```python
from build123d import *

# Parameters (mm, degrees)
SKETCH1_W                         = 78
SKETCH1_H                         = 60
BOSS_EXTRUDE1_DEPTH               = 9.3
TAP_DRILL_FOR_M5_TAP1_D           = 5.2
TAP_DRILL_FOR_M5_TAP1_DEPTH       = 46
TAP_DRILL_FOR_M5_TAP1_CSINK_D     = 6
TAP_DRILL_FOR_M5_TAP1_CSINK_ANGLE = 90
TAP_DRILL_FOR_M5_TAP1_TIP         = 1.562237609
SKETCH4_W                         = 61.6
SKETCH4_H                         = 60
CUT_EXTRUDE1_DEPTH                = 5.3
CHAMFER1_SIZE                     = 3
CUT_EXTRUDE2_DEPTH                = 4
FILLET1_R                         = 1
FILLET2_R                         = 1
SKETCH7_W                         = 8
SKETCH7_H                         = 20
BOSS_EXTRUDE2_DEPTH               = 5.3
SKETCH8_R                         = 1.75
CUT_EXTRUDE3_DEPTH                = 5.3


with BuildPart() as part:
    # Sketch1 → Boss-Extrude1 (new body)
    with BuildSketch(Plane(origin=(0, 0, 0), x_dir=(1, 0, 0), z_dir=(0, 1, 0))):
        Rectangle(SKETCH1_W, SKETCH1_H)
    extrude(amount=BOSS_EXTRUDE1_DEPTH)

    # Tap Drill for M5 Tap1
    with Locations(Plane(origin=(-36, 9.3, -15), x_dir=(0, 0, 1), z_dir=(0, 1, 0))):
        with Locations((0, 0), (30, 0), (30, 72), (0, 72)):
            CounterSinkHole(TAP_DRILL_FOR_M5_TAP1_D / 2, TAP_DRILL_FOR_M5_TAP1_CSINK_D / 2, depth=TAP_DRILL_FOR_M5_TAP1_DEPTH, counter_sink_angle=TAP_DRILL_FOR_M5_TAP1_CSINK_ANGLE)
            with Locations((0, 0, -(TAP_DRILL_FOR_M5_TAP1_DEPTH + TAP_DRILL_FOR_M5_TAP1_TIP / 2))):  # 118° drill point
                Cone(0, TAP_DRILL_FOR_M5_TAP1_D / 2, TAP_DRILL_FOR_M5_TAP1_TIP, mode=Mode.SUBTRACT)

    # Sketch4 → Cut-Extrude1 (cut)
    with BuildSketch(Plane(origin=(0, 9.3, 0), x_dir=(1, 0, 0), z_dir=(0, 1, 0))):
        Rectangle(SKETCH4_W, SKETCH4_H)
    extrude(amount=-CUT_EXTRUDE1_DEPTH, mode=Mode.SUBTRACT)

    # Chamfer1
    chamfer1_edges = [part.edges().sort_by_distance(p)[0] for p in [
        (39, 4.65, 30),
        (-39, 4.65, 30),
        (-39, 4.65, -30),
        (39, 4.65, -30),
    ]]
    chamfer(chamfer1_edges, length=CHAMFER1_SIZE)

    # Sketch6 → Cut-Extrude2 (cut)
    with BuildSketch(Plane(origin=(0, 9.3, 0), x_dir=(1, 0, 0), z_dir=(0, 1, 0))):
        with BuildLine():
            Line((-39.66, 19.25), (-36, 19.25))
            ThreePointArc((-36, 19.25), (-31.75, 15), (-36, 10.75))
            Line((-36, 10.75), (-39.66, 10.75))
            ThreePointArc((-39.66, 10.75), (-43.91, 15), (-39.66, 19.25))
        make_face()
        with BuildLine():
            Line((-39.66, -19.25), (-36, -19.25))
            ThreePointArc((-36, -19.25), (-31.75, -15), (-36, -10.75))
            Line((-36, -10.75), (-39.66, -10.75))
            ThreePointArc((-39.66, -10.75), (-43.91, -15), (-39.66, -19.25))
        make_face()
        with BuildLine():
            Line((39.66, 19.25), (36, 19.25))
            ThreePointArc((36, 19.25), (31.75, 15), (36, 10.75))
            Line((36, 10.75), (39.66, 10.75))
            ThreePointArc((39.66, 10.75), (43.91, 15), (39.66, 19.25))
        make_face()
        with BuildLine():
            Line((39.66, -10.75), (36, -10.75))
            ThreePointArc((36, -10.75), (31.75, -15), (36, -19.25))
            Line((36, -19.25), (39.66, -19.25))
            ThreePointArc((39.66, -19.25), (43.91, -15), (39.66, -10.75))
        make_face()
    extrude(amount=-CUT_EXTRUDE2_DEPTH, mode=Mode.SUBTRACT)

    # Fillet1
    fillet1_edges = [part.edges().sort_by_distance(p)[0] for p in [
        (-39, 4.65, 27),
        (-39, 4.65, -27),
        (36, 4.65, -30),
        (-36, 4.65, -30),
        (39, 4.65, 27),
        (39, 4.65, -27),
        (-36, 4.65, 30),
        (36, 4.65, 30),
    ]]
    fillet(fillet1_edges, radius=FILLET1_R)

    # Fillet2
    fillet2_edges = [part.edges().sort_by_distance(p)[0] for p in [
        (39, 7.3, -10.75),
        (39, 7.3, -19.25),
        (39, 7.3, 19.25),
        (39, 7.3, 10.75),
        (-39, 7.3, -19.25),
        (-39, 7.3, -10.75),
        (-39, 7.3, 19.25),
        (-39, 7.3, 10.75),
    ]]
    fillet(fillet2_edges, radius=FILLET2_R)

    # Sketch7 → Boss-Extrude2 (add)
    with BuildSketch(Plane(origin=(0, 4, 0), x_dir=(1, 0, 0), z_dir=(0, 1, 0))):
        with Locations((-26.8, -20)):
            Rectangle(SKETCH7_W, SKETCH7_H)
        with Locations((26.8, -20)):
            Rectangle(SKETCH7_W, SKETCH7_H)
    extrude(amount=BOSS_EXTRUDE2_DEPTH)

    # Sketch8 → Cut-Extrude3 (cut)
    with BuildSketch(Plane(origin=(0, 9.3, 0), x_dir=(1, 0, 0), z_dir=(0, 1, 0))):
        with Locations((30.8, -8.25)):
            Circle(SKETCH8_R)
        with Locations((-30.8, -8.25)):
            Circle(SKETCH8_R)
    extrude(amount=-CUT_EXTRUDE3_DEPTH, mode=Mode.SUBTRACT)


solid = part.part
```
Check sheet for the modelled part. Datum: model origin and axes. Units: mm. A direction names the side the tool comes from. Round coordinates to 2 decimals unless told otherwise and drop trailing zeros. Loops run counter-clockwise (first coordinate to the right, second up) from the corner with the lowest first, then second, coordinate; pieces in that order, holes last. Notation, with made-up numbers: (11, 56.5) - (63, 56.5) arc R23 cw to (63, 94.5) - close; hole circle Ø8 at (-18.5, 67). An arc over 180 degrees is marked (long way). Answer as a JSON object with one key per item and string values. Group by question number.
Q1. Set-up check for faces 4 (the face through (-34.6, 5.3, 12.6)), 5 (the face through (37, 7, -10.75)), 6 (the face through (-22.8, 7, 20)): record each of +Z, -Z, +X, -X, +Y, -Y from which the full face is reachable in a straight line by a thin tool's end or side.
Q2. Sectioned sample at D-D, the plane x = -10. Enter the section's corners in (y, z).
Q3. Mould release check, pull along Z, two halves, no side actions. Record for faces 1 (the face through (-0.5, 3.6, 30)), 2 (the face through (22.8, 7, 20)), 3 (the face through (33, 5.3, 15)): released by +Z, released by -Z, zero draft, split by the parting line, or undercut.
Q4. Sectioned sample at A-A, the plane z = 15. Enter the section's corners in (x, y).
Q5. Sectioned sample at C-C, the plane z = -22.5. Enter the section's corners in (x, y).
Q6. Gauge pin test, flat ends, axial feed: P1, Ø4, axis at x = -13, z = -21.5, coming from the -Y side; P2, Ø1, axis at x = 37.5, y = 7.5, coming from the -Z side; P3, Ø7, axis at x = -36, z = 15, coming from the +Y side; P4, Ø1.6, axis at x = 37, y = 7, coming from the +Z side. Record the tip position at first contact, or that the pin passes through.
Q7. Sectioned sample at B-B, the plane y = 1.25. Enter the section's corners in (x, z).
Q8. Scan lines: line 1 along X through (y, z) = (2.25, -15); line 2 along X through (y, z) = (7.5, -22.5); line 3 along Y through (x, z) = (11.5, 11.5). Record each from-to range of solid material in increasing order. Write a range as [from, to].
Solution:
{
 "1": {"face 4": "-X, +Y", "face 5": "+X, +Y", "face 6": "+Z, -Z, +Y"},
 "2": {"outline": "(0, -30) - (4, -30) - (4, 30) - (0, 30) - close"},
 "3": {"face 1": "released by +Z", "face 2": "zero draft", "face 3": "undercut"},
 "4": {"outline": "(-39, 0) - (-38.6, 0) - (-38.6, 5.3) - (-39, 5.3) - close; (-33.4, 0) - (33.4, 0) - (33.4, 5.3) - (31.75, 5.3) - (31.75, 9.3) - (22.8, 9.3) - (22.8, 4) - (-22.8, 4) - (-22.8, 9.3) - (-31.75, 9.3) - (-31.75, 5.3) - (-33.4, 5.3) - close; (38.6, 0) - (39, 0) - (39, 5.3) - (38.6, 5.3) - close"},
 "5": {"outline": "(-39, 0) - (39, 0) - (39, 9.3) - (30.8, 9.3) - (30.8, 4) - (-30.8, 4) - (-30.8, 9.3) - (-39, 9.3) - close"},
 "6": {"P1": "stops at y = 0", "P2": "stops at z = -29", "P3": "stops at y = 5.3", "P4": "stops at z = 29.79"},
 "7": {"outline": "(-39, -26.59) arc R1 ccw to (-38.71, -27.29) - (-36.29, -29.71) arc R1 ccw to (-35.59, -30) - (35.59, -30) arc R1 ccw to (36.29, -29.71) - (38.71, -27.29) arc R1 ccw to (39, -26.59) - (39, 26.59) arc R1 ccw to (38.71, 27.29) - (36.29, 29.71) arc R1 ccw to (35.59, 30) - (-35.59, 30) arc R1 ccw to (-36.29, 29.71) - (-38.71, 27.29) arc R1 ccw to (-39, 26.59) - close; hole circle Ø5.2 at (-36, -15); hole circle Ø5.2 at (-36, 15); hole circle Ø5.2 at (36, -15); hole circle Ø5.2 at (36, 15)"},
 "8": {"line 1": "x = [-39, -38.6], [-33.4, 33.4], [38.6, 39]", "line 2": "x = [-39, -30.8], [30.8, 39]", "line 3": "y = [0, 4]"}
}
